Part model, mm, in its own coordinate system. A direction names the side the tool comes from. Give positions to 0.01 mm unless a question says otherwise; leave off trailing zeros. Write each loop counter-clockwise with the first axis right and the second up, starting at its lowest first coordinate (ties: lowest second). Pieces come first, ordered by that corner, then holes. Notation, with made-up numbers: (79.25, 84) - (128.25, 84) arc R9 ccw to (128.25, 94) - close; hole circle Ø10 at (24, 14). An arc over 180 degrees is marked (long way). Answer as a JSON object with one key per item and string values. Group by question number.
```python
from build123d import *

# Parameters (mm, degrees)
BOSS_EXTRUDE1_DEPTH = 115
SKETCH3_R           = 55
BOSS_EXTRUDE2_DEPTH = 40
CUT_EXTRUDE2_REACH  = 312.524
SKETCH2_R           = 30
CUT_EXTRUDE3_DEPTH  = 5


with BuildPart() as part:
    # Sketch1 → Boss-Extrude1 (new, symmetric)
    with BuildSketch(Plane.XY):
        Polygon((80, 0), (-80, 0), (-80, 240), (-50, 240), (-50, 20), (50, 20), (50, 240), (80, 240), align=None)
    extrude(amount=BOSS_EXTRUDE1_DEPTH, both=True)

    # Sketch3 → Boss-Extrude2 (add)
    with BuildSketch(Plane.XZ):
        with Locations(Location((0, 0, 0), (0, 0, 270))):
            Circle(SKETCH3_R)
    extrude(amount=BOSS_EXTRUDE2_DEPTH)

    # Cut-Extrude2: up to this face of the body (flat: up to its plane)
    cut_extrude2_end = Plane(part.part.faces().sort_by_distance((80, 120, 0))[0])
    # Sketch2 → Cut-Extrude2 (cut, up to the picked face)
    with BuildSketch(Plane.ZY.offset(80), mode=Mode.PRIVATE) as cut_extrude2_sk1:
        with BuildLine():
            ThreePointArc((-75, 165), (-53.033008792, 218.033008386), (-5.74e-07, 240))
            Line((-5.74e-07, 240), (-115, 240))
            Line((-115, 240), (-115, 20))
            Line((-115, 20), (-75, 165))
        make_face()
    cut_extrude2_tool1 = split(extrude(cut_extrude2_sk1.sketch, amount=-CUT_EXTRUDE2_REACH, mode=Mode.PRIVATE), bisect_by=cut_extrude2_end, keep=Keep.BOTH, mode=Mode.PRIVATE)
    # Sketch2 → Cut-Extrude2 (cut, up to the picked face)
    with BuildSketch(Plane.ZY.offset(80), mode=Mode.PRIVATE) as cut_extrude2_sk2:
        with BuildLine():
            ThreePointArc((-5.74e-07, 240), (53.033008386, 218.033008792), (75, 165))
            Line((75, 165), (115, 20))
            Line((115, 20), (115, 240))
            Line((115, 240), (-5.74e-07, 240))
        make_face()
    cut_extrude2_tool2 = split(extrude(cut_extrude2_sk2.sketch, amount=-CUT_EXTRUDE2_REACH, mode=Mode.PRIVATE), bisect_by=cut_extrude2_end, keep=Keep.BOTH, mode=Mode.PRIVATE)
    # Sketch2 → Cut-Extrude2 (cut, up to the picked face)
    with BuildSketch(Plane.ZY.offset(80), mode=Mode.PRIVATE) as cut_extrude2_sk3:
        with Locations((0, 165)):
            Circle(SKETCH2_R)
    cut_extrude2_tool3 = split(extrude(cut_extrude2_sk3.sketch, amount=-CUT_EXTRUDE2_REACH, mode=Mode.PRIVATE), bisect_by=cut_extrude2_end, keep=Keep.BOTH, mode=Mode.PRIVATE)
    add(cut_extrude2_tool1.solids().sort_by(Axis((-80, 171.000425, -91.477903), (1, 0, 0)))[0], mode=Mode.SUBTRACT)
    add(cut_extrude2_tool2.solids().sort_by(Axis((-80, 171.000425, 91.477903), (1, 0, 0)))[0], mode=Mode.SUBTRACT)
    add(cut_extrude2_tool3.solids().sort_by(Axis((-80, 165, 0), (1, 0, 0)))[0], mode=Mode.SUBTRACT)

    # Sketch4 → Cut-Extrude3 (cut)
    with BuildSketch(Plane.ZY.offset(80)):
        with BuildLine():
            Line((15, 108.832847002), (15, 33.352154436))
            ThreePointArc((15, 33.352154436), (0, 18.352154436), (-15, 33.352154436))
            Line((-15, 33.352154436), (-15, 108.832847002))
            ThreePointArc((-15, 108.832847002), (0, 123.832847002), (15, 108.832847002))
        make_face()
    cut_extrude3 = extrude(amount=-CUT_EXTRUDE3_DEPTH, mode=Mode.SUBTRACT)

    # Mirror1: Cut-Extrude3 across plane
    add(cut_extrude3.mirror(Plane(origin=(0, 0, 0), x_dir=(0, 0, 1), z_dir=(1, 0, 0))), mode=Mode.SUBTRACT)


solid = part.part
```
1) Saw through at B-B (x = -63). List the corners of the cut face in (y, z), and give its area (3 significant figures).
2) Two-plate mould, pull along Y, no slides. Class faces 4 (the cylindrical face through (77.535, 18.356, 0.33)), 5 (the cylindrical face through (-65.21, 239.98, -1.65)), 6 (the flat face through (19, 0, 53)), 7 (the cylindrical face through (-48.794, -19.72, -25.379)): +Y half, -Y half, draft (parallel to the pull), parting line (faces both ways), or undercut.
3) Which spindle directions (+Z, -Z, +X, -X, +Y, -Y) get a long thin tool onto all of the face, cutting with end or side? Do faces 1 (the flat face through (75, 72, 0)), 2 (the cylindrical face through (-77.54, 123.83, -0.33)), 3 (the flat face through (-1, 20, 2)). Say none if no direction does.
4) Drill centre lines: line 1 along Y through (x, z) = (66, 0); line 2 along X through (y, z) = (44, -22.5); line 3 along Y through (x, z) = (-46, 97.5). Where is each one in solid material? Low to high. Write a range as from..to.
5) Saw through at C-C (y = 43). List the corners of the cut face in (x, z), and give its area (3 significant figures).
6) Saw through at D-D (x = 0). List the corners of the cut face in (y, z), and give its area (3 significant figures).
7) Drop flat-ended pins along their axis: P1, Ø5.5, axis at x = -76.5, y = 74, coming from the -Z side; P2, Ø1.5, axis at x = 77, y = 63.5, coming from the -Z side; P3, Ø12, axis at x = -5, z = 74.5, coming from the -Y side. Give the stop position or say it passes through.
8) Saw through at A-A (z = 0). List the corners of the cut face in (x, y).
Checks:
{
 "1": {"outline": "(0, -115) - (20, -115) - (165, -75) arc R75 ccw to (165, 75) - (20, 115) - (0, 115) - close; hole circle Ø60 at (165, 0)", "area": "38,200 mm2"},
 "2": {"face 4": "undercut", "face 5": "+Y half", "face 6": "-Y half", "face 7": "draft"},
 "3": {"face 1": "+X", "face 2": "-X", "face 3": "+Z, -Z, +Y"},
 "4": {"line 1": "0..135, 195..240", "line 2": "-80..-50, 50..80", "line 3": "0..20"},
 "5": {"outline": "(-80, -108.66) - (-50, -108.66) - (-50, 108.66) - (-80, 108.66) - (-80, 15) - (-75, 15) - (-75, -15) - (-80, -15) - close; (50, -108.66) - (80, -108.66) - (80, -15) - (75, -15) - (75, 15) - (80, 15) - (80, 108.66) - (50, 108.66) - close", "area": "12,700 mm2"},
 "6": {"outline": "(-40, -55) - (0, -55) - (0, -115) - (20, -115) - (20, 115) - (0, 115) - (0, 55) - (-40, 55) - close", "area": "9,000 mm2"},
 "7": {"P1": "z = -100.86", "P2": "z = -103.21", "P3": "y = 0"},
 "8": {"outline": "(-80, 0) - (-55, 0) - (-55, -40) - (55, -40) - (55, 0) - (80, 0) - (80, 18.35) - (75, 18.35) - (75, 123.83) - (80, 123.83) - (80, 135) - (50, 135) - (50, 20) - (-50, 20) - (-50, 135) - (-80, 135) - (-80, 123.83) - (-75, 123.83) - (-75, 18.35) - (-80, 18.35) - close; (-80, 195) - (-50, 195) - (-50, 240) - (-80, 240) - close; (50, 195) - (80, 195) - (80, 240) - (50, 240) - close"}
}
